Can you work these out from the drawing? Everything is in mm from the part's minimum corner. Give positions to 0.01 mm unless a question says otherwise; leave off trailing zeros. Order: outer loops, then holes, each group sorted by start corner. A loop starts at its lowest first (then second) coordinate and runs counter-clockwise, first axis right, second up. Notation, with made-up numbers: (15, 19.5) - (59, 19.5) arc R30 ccw to (59, 41.5) - close; hole circle Ø3 at (71.5, 43). An arc over 180 degrees is marked (long way). Answer as a JSON object with one key per item and string values.
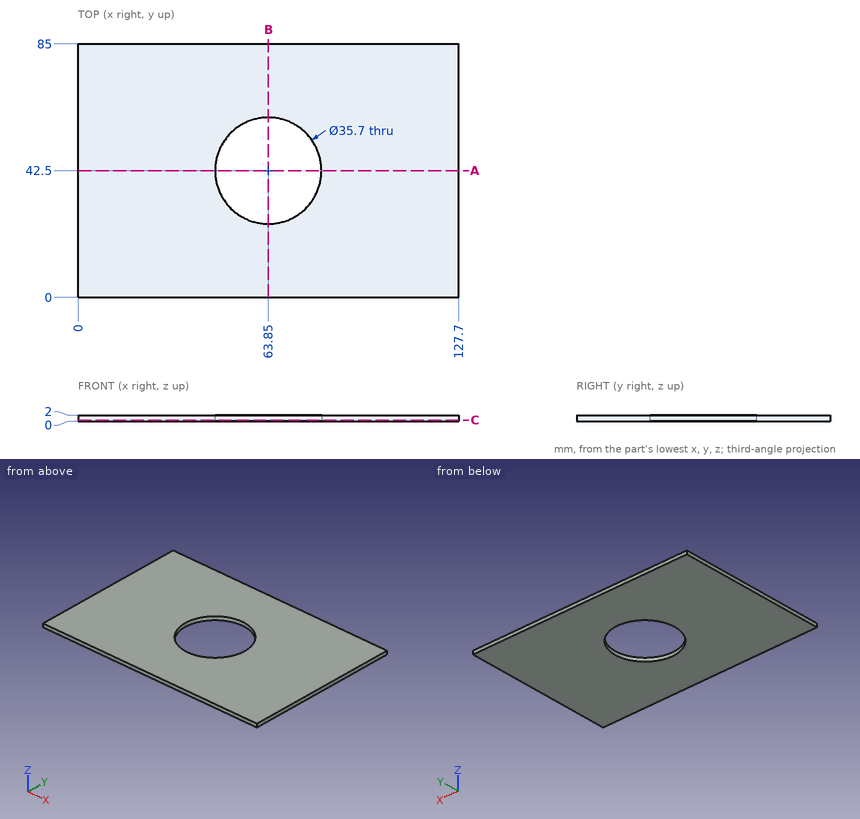
Q1. I'm going to push a flat-ended pin straight in: pin 1 Ø1.5 at (x, y) = (45.5, 29.5) entering from -Z. Where does the tip first touch, or does it pass through?
Recorded:
{"pin 1": "stops at z = 0"}
Q2. If we section it at A-A, the plane y = 42.5: Please give me the cut outline in (x, z), then the cut area to 3 significant figures.
Recorded:
{"outline": "(0, 0) - (46, 0) - (46, 2) - (0, 2) - close; (81.7, 0) - (127.7, 0) - (127.7, 2) - (81.7, 2) - close", "area": "184 mm^2"}
Q3. If we section it at B-B, the plane x = 63.85: Please give me the cut outline in (y, z), then the cut area to 3 significant figures.
Recorded:
{"outline": "(0, 0) - (24.65, 0) - (24.65, 2) - (0, 2) - close; (60.35, 0) - (85, 0) - (85, 2) - (60.35, 2) - close", "area": "98.6 mm^2"}
Q4. If we section it at C-C, the plane z = 0.4: Please give me the cut outline in (x, y).
Recorded:
{"outline": "(0, 0) - (127.7, 0) - (127.7, 85) - (0, 85) - close; hole circle Ø35.7 at (63.85, 42.5)"}
Q5. I need wall thicknesses on L1, parallel to Y at x = 63.85, z = 1.25; L2, parallel to X at y = 40.5, z = 1.8; L3, parallel to X at y = 33, z = 1.45. Which ranges of each line are inside material? Lowest first, please.
Recorded:
{"L1": "y = 0 to 24.65, 60.35 to 85", "L2": "x = 0 to 46.11, 81.59 to 127.7", "L3": "x = 0 to 48.74, 78.96 to 127.7"}
